Could you check a few things on this drawing? It's one solid part, dimensions in mm from its lowest x, y, z. Give positions to 0.01 mm unless a question says otherwise; leave off trailing zeros. Loops run counter-clockwise (first coordinate to the right, second up) from the corner with the lowest first, then second, coordinate; pieces in that order, holes last.
1. For P1, Ø2.5, axis at y = 57.5, z = 2.5, coming from the -X side; P2, Ø1.5, axis at x = 85, z = 3.5, coming from the -Y side; P3, Ø2.5, axis at x = 40, z = 1.5, coming from the -Y side; P4, Ø1.4, axis at x = 76, z = 4, coming from the -Y side, each with a flat end and sliding along its axis, tell me the tip position at first contact or that it passes through.
2. Imagine slicing it at C-C (x = 82). List the corners of the cut face in (y, z) for me.
3. Imagine slicing it at D-D (y = 132). List the corners of the cut face in (x, z) for me, plus the area to 3 significant figures.
4. Imagine slicing it at B-B (z = 2.15). List the corners of the cut face in (x, y) for me, plus the area to 3 significant figures.
5. Imagine slicing it at A-A (y = 43.5). List the corners of the cut face in (x, z) for me.
6. I need wall thicknesses on line 1 along X through (y, z) = (51, 2.8); line 2 along X through (y, z) = (66.5, 3.7); line 3 along Y through (x, z) = (103, 3.3). Which ranges of each line are inside material? Lowest first, please.
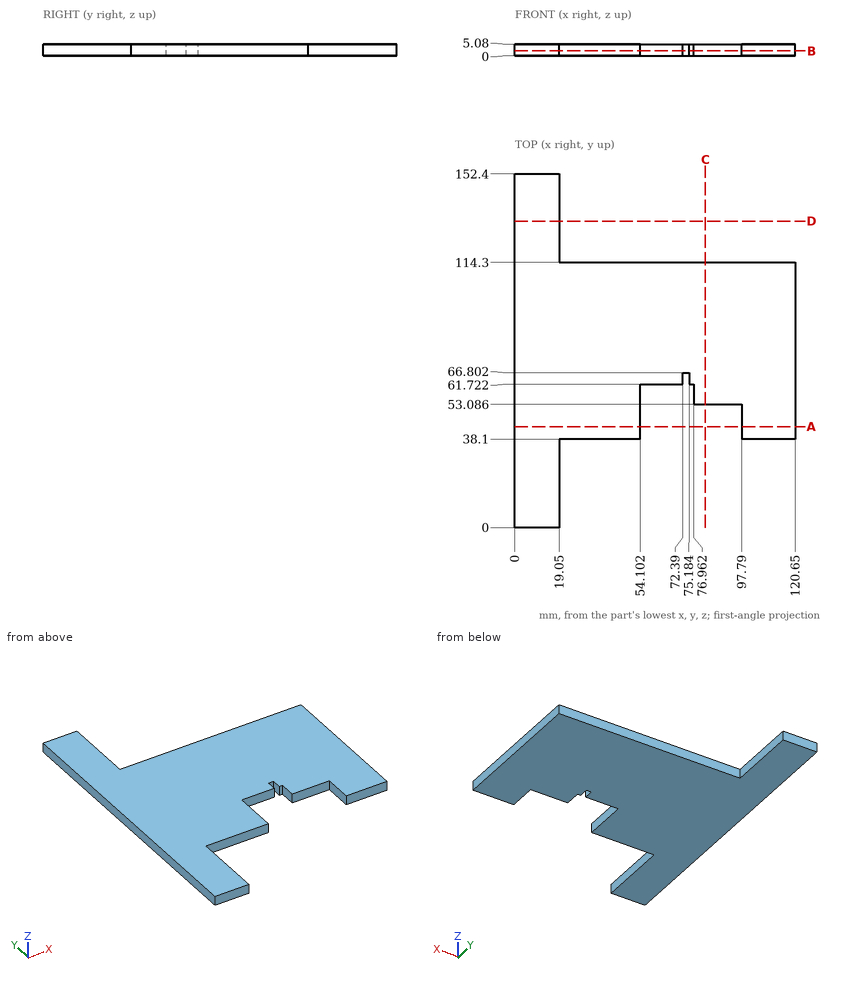
Derived:
1. P1: stops at x = 0
1. P2: stops at y = 53.09
1. P3: stops at y = 38.1
1. P4: stops at y = 61.72
2. outline: (53.09, 0) - (114.3, 0) - (114.3, 5.08) - (53.09, 5.08) - close
3. outline: (0, 0) - (19.05, 0) - (19.05, 5.08) - (0, 5.08) - close
3. area: 96.8 mm2
4. outline: (0, 0) - (19.05, 0) - (19.05, 38.1) - (54.1, 38.1) - (54.1, 61.72) - (72.39, 61.72) - (72.39, 66.8) - (75.18, 66.8) - (75.18, 61.72) - (76.96, 61.72) - (76.96, 53.09) - (97.79, 53.09) - (97.79, 38.1) - (120.65, 38.1) - (120.65, 114.3) - (19.05, 114.3) - (19.05, 152.4) - (0, 152.4) - close
4. area: 9,780 mm2
5. outline: (0, 0) - (54.1, 0) - (54.1, 5.08) - (0, 5.08) - close; (97.79, 0) - (120.65, 0) - (120.65, 5.08) - (97.79, 5.08) - close
6. line 1: x = 0 to 54.1, 97.79 to 120.65
6. line 2: x = 0 to 72.39, 75.18 to 120.65
6. line 3: y = 38.1 to 114.3
